For this review, take the finished solid that the model builds, in its own axes (mm). A direction names the side the tool comes from. Coordinates: 2 decimals unless noted, no trailing zeros. Write each loop counter-clockwise with the first axis right and the second up, starting at its lowest first coordinate (ties: lowest second). Pieces come first, ordered by that corner, then holes.
```python
from build123d import *

# Parameters (mm, degrees)
SKETCH035_R  = 2.2
PAD019_DEPTH = 2
SKETCH036_W  = 28
SKETCH036_H  = 6
PAD021_DEPTH = 2.5
SKETCH037_W  = 27
SKETCH037_H  = 20
SKETCH038_W  = 16
SKETCH038_H  = 20
FILLET006_R  = 2
SKETCH041_W  = 16
SKETCH041_H  = 20
PAD022_DEPTH = 11.001
SKETCH039_R  = 1.75
PAD023_DEPTH = 6.5
FILLET004_R  = 11
FILLET005_R  = 4.5
FILLET007_R  = 4.5


with BuildPart() as part:
    # Sketch035 → Pad019 (new body)
    with BuildSketch(Plane.XY):
        with BuildLine():
            Line((-25.5, 10), (25.5, 10))
            ThreePointArc((27.5, 8), (26.914214, 9.414214), (25.5, 10))
            Line((27.5, 8), (27.5, -8))
            ThreePointArc((25.5, -10), (26.914214, -9.414214), (27.5, -8))
            Line((25.5, -10), (-25.5, -10))
            ThreePointArc((-27.5, -8), (-26.914214, -9.414214), (-25.5, -10))
            Line((-27.5, -8), (-27.5, 8))
            ThreePointArc((-25.5, 10), (-26.914214, 9.414214), (-27.5, 8))
        make_face()
        with Locations((-20, 0)):
            Circle(SKETCH035_R, mode=Mode.SUBTRACT)
        with Locations((20, 0)):
            Circle(SKETCH035_R, mode=Mode.SUBTRACT)
    extrude(amount=-PAD019_DEPTH)

    # Sketch036 → Pad021 (join)
    with BuildSketch(Plane(origin=(0, 0, -2), x_dir=(1, 0, 0), z_dir=(0, 0, -1))):
        Rectangle(SKETCH036_W, SKETCH036_H)
    extrude(amount=PAD021_DEPTH)

    # Sketch037 → AdditiveLoft001 section 0
    with BuildSketch(Plane.XY):
        Rectangle(SKETCH037_W, SKETCH037_H)
    # Sketch038 → AdditiveLoft001 section 1
    with BuildSketch(Plane.XY.offset(35)):
        Rectangle(SKETCH038_W, SKETCH038_H)
    loft()

    # Fillet006
    fillet006_edges = [part.edges().sort_by_distance(p)[0] for p in [
        (-13.5, 0, 0),
        (13.5, 0, 0),
    ]]
    fillet(fillet006_edges, radius=FILLET006_R)

    # Sketch041 → Pad022 (join)
    with BuildSketch(Plane.XY.offset(35)):
        Rectangle(SKETCH041_W, SKETCH041_H)
    extrude(amount=PAD022_DEPTH)

    # Sketch039 → Pad023 (join)
    with BuildSketch(Plane(origin=(0, -10, 35), x_dir=(-1, 0, 0), z_dir=(0, 0, 1))):
        with BuildLine():
            Line((8, 0), (-8, 0))
            Line((-8, 0), (-8, 13))
            ThreePointArc((8, 13), (0, 21), (-8, 13))
            Line((8, 13), (8, 0))
        make_face()
        with Locations((0, 13)):
            Circle(SKETCH039_R, mode=Mode.SUBTRACT)
    extrude(amount=PAD023_DEPTH)

    # Fillet004
    fillet004_edges = [part.edges().sort_by_distance(p)[0] for p in [
        (0, 10, 46.001),
    ]]
    fillet(fillet004_edges, radius=FILLET004_R)

    # Fillet005
    fillet005_edges = [part.edges().sort_by_distance(p)[0] for p in [
        (0, -10, 41.5),
        (0, -10, 35),
    ]]
    fillet(fillet005_edges, radius=FILLET005_R)

    # Fillet007
    fillet007_edges = [part.edges().sort_by_distance(p)[0] for p in [
        (0, -10, 46.001),
    ]]
    fillet(fillet007_edges, radius=FILLET007_R)


solid = part.part
```
Q1. Add section B-B (y = 0). State the section outline as (x, z) points.
Ans:
outline: (-27.5, -2) - (-22.2, -2) - (-22.2, 0) - (-27.5, 0) - close; (-17.8, -2) - (-14, -2) - (-14, -4.5) - (14, -4.5) - (14, -2) - (17.8, -2) - (17.8, 0) - (15.21, 0) arc R2 cw to (13.23, 1.69) - (8, 35) - (8, 45.96) - (-8, 45.96) - (-8, 35) - (-13.23, 1.69) arc R2 cw to (-15.21, 0) - (-17.8, 0) - close; (22.2, -2) - (27.5, -2) - (27.5, 0) - (22.2, 0) - close
Q2. Tool access review of faces 1 (the flat face through (0, 3, -3)), 2 (the flat face through (-14, 0, -3)), 3 (the flat face through (14, 0, -3)), 4 (the flat face through (0, -21, 41.5)): name each direction out of +Z, -Z, +X, -X, +Y, -Y from which nothing blocks a thin tool from reaching the whole face with its end or side.
Ans:
face 1: -Z, +X, -X, +Y
face 2: -Z, -X, +Y, -Y
face 3: -Z, +X, +Y, -Y
face 4: +Z, +X, -X, -Y
Q3. Clearance check with flat-ended pins moving along their axes: pin 1 Ø3 at (y, z) = (0.5, -2.5) entering from -X; pin 2 Ø13.5 at (x, y) = (-23, -3.5) entering from +Z; pin 3 Ø12 at (y, z) = (-13, 41) entering from +X; pin 4 Ø13.5 at (x, y) = (20.5, -2.5) entering from +Z. State where each tip first meets the part, or that it passes through.
Ans:
pin 1: stops at x = -27.5
pin 2: stops at z = 0
pin 3: stops at x = 8
pin 4: stops at z = 0.63
Q4. Draft analysis for pull direction X (two halves, no side actions). For faces 5 (the flat face through (0, -4, 46.001)), 6 (the cylindrical face through (22.032, -0.843, -0.986)), 7 (the cylindrical face through (-13.926, 0.14, 0.467)), 8 (the flat face through (10.58, 0.3, 18.58)), state which applies: +X half, -X half, draft (parallel to the pull), parting line (faces both ways), or undercut.
Ans:
face 5: draft
face 6: undercut
face 7: -X half
face 8: +X half
Q5. For probe 1 along X at (y, z) = (-23, 38); probe 2 along Z at (x, y) = (-18.5, 2); probe 3 along Z at (x, y) = (-5.5, -4), list the stretches that pass through material, from the lowest coordinate up.
Ans:
probe 1: x = -8 to -1.75, 1.75 to 8
probe 2: z = -2 to 0
probe 3: z = -2 to 46
Q6. Add section A-A (x = 20). State the section outline as (y, z) points, then the cut area to 3 significant figures.
Ans:
outline: (-10, -2) - (-2.2, -2) - (-2.2, 0) - (-10, 0) - close; (2.2, -2) - (10, -2) - (10, 0) - (2.2, 0) - close
area: 31.2 mm2
Q7. Add section C-C (z = 10.5). State the section outline as (x, y) points, then the cut area to 3 significant figures.
Ans:
outline: (-11.85, -10) - (11.85, -10) - (11.85, 10) - (-11.85, 10) - close
area: 474 mm2
Q8. Add section D-D (y = -19.5). State the section outline as (x, z) points, then the cut area to 3 significant figures.
Ans:
outline: (-8, 35) - (8, 35) - (8, 41.5) - (-8, 41.5) - close
area: 104 mm2
